```python
from build123d import *

# Parameters (mm, degrees)
SKETCH1_R           = 76.2
BOSS_EXTRUDE1_DEPTH = 40
BOSS_EXTRUDE2_DEPTH = 30
CIRPATTERN1_COUNT   = 10
BOSS_EXTRUDE3_DEPTH = 30
CIRPATTERN2_COUNT   = 10
SKETCH4_R           = 7.9375
CUT_EXTRUDE1_DEPTH  = 41
CUT_EXTRUDE2_DEPTH  = 41
CIRPATTERN3_COUNT   = 8
FILLET4_R           = 5
FILLET5_R           = 5


with BuildPart() as part:
    # Sketch1 → Boss-Extrude1 (new body)
    with BuildSketch(Plane(origin=(0, 0, 0), x_dir=(1, 0, 0), z_dir=(0, 1, 0))):
        Circle(SKETCH1_R)
    extrude(amount=BOSS_EXTRUDE1_DEPTH)

    # Sketch2 → Boss-Extrude2 (add)
    with BuildSketch(Plane(origin=(0, 40, 0), x_dir=(1, 0, 0), z_dir=(0, 1, 0))):
        with BuildLine():
            Line((0, 86.2), (0, 76.2))
            ThreePointArc((0, 76.2), (2.860964701, 76.146272929), (5.717894985, 75.98516748))
            Line((5.717894985, 75.98516748), (2, 86.2))
            Line((2, 86.2), (0, 86.2))
        make_face()
        with BuildLine():
            ThreePointArc((-5.717894985, 75.98516748), (-2.860964701, 76.146272929), (0, 76.2))
            Line((0, 76.2), (0, 86.2))
            Line((0, 86.2), (-2, 86.2))
            Line((-2, 86.2), (-5.717894985, 75.98516748))
        make_face()
    boss_extrude2 = extrude(amount=-BOSS_EXTRUDE2_DEPTH)

    # CirPattern1: Boss-Extrude2 ×10 about axis
    cirpattern1_axis = Axis((0, 0, -0.338660651), (0, 1, 0))
    for i in range(1, CIRPATTERN1_COUNT):
        add(boss_extrude2.rotate(cirpattern1_axis, i * 360 / CIRPATTERN1_COUNT))

    # Sketch3 → Boss-Extrude3 (add)
    with BuildSketch(Plane.XZ):
        with BuildLine():
            Line((24.811616962, 82.515457643), (17.980532935, 74.048230468))
            ThreePointArc((17.980532935, 74.048230468), (20.820375524, 73.300422666), (23.629294983, 72.44374658))
            Line((23.629294983, 72.44374658), (26.73025233, 81.950799937))
            Line((26.73025233, 81.950799937), (24.811616962, 82.515457643))
        make_face()
        with BuildLine():
            Line((26.73025233, 81.950799937), (23.629294983, 72.44374658))
            ThreePointArc((23.629294983, 72.44374658), (26.423605423, 71.471904105), (29.178084826, 70.392324624))
            Line((29.178084826, 70.392324624), (28.648887698, 81.386142232))
            Line((28.648887698, 81.386142232), (26.73025233, 81.950799937))
        make_face()
    boss_extrude3 = extrude(amount=-BOSS_EXTRUDE3_DEPTH)

    # CirPattern2: Boss-Extrude3 ×10 about axis
    cirpattern2_axis = Axis((0.107387074, 0, 0.328898849), (0, 1, 0))
    for i in range(1, CIRPATTERN2_COUNT):
        add(boss_extrude3.rotate(cirpattern2_axis, i * 360 / CIRPATTERN2_COUNT))

    # Sketch4 → Cut-Extrude1 (cut, through all)
    with BuildSketch(Plane(origin=(0, 40, 0), x_dir=(1, 0, 0), z_dir=(0, 1, 0))):
        Circle(SKETCH4_R)
    extrude(amount=-CUT_EXTRUDE1_DEPTH, mode=Mode.SUBTRACT)

    # Sketch5 → Cut-Extrude2 (cut, through all)
    with BuildSketch(Plane(origin=(0, 40, 0), x_dir=(1, 0, 0), z_dir=(0, 1, 0))):
        with BuildLine():
            ThreePointArc((15, 62.217360921), (0, 64), (-15, 62.217360921))
            Line((-15, 62.217360921), (-5, 19.364916731))
            ThreePointArc((-5, 19.364916731), (0, 20), (5, 19.364916731))
            Line((5, 19.364916731), (15, 62.217360921))
        make_face()
    cut_extrude2 = extrude(amount=-CUT_EXTRUDE2_DEPTH, mode=Mode.SUBTRACT)

    # CirPattern3: Cut-Extrude2 ×8 about axis
    cirpattern3_axis = Axis((0, 0, 0), (0, 1, 0))
    for i in range(1, CIRPATTERN3_COUNT):
        add(cut_extrude2.rotate(cirpattern3_axis, i * 360 / CIRPATTERN3_COUNT), mode=Mode.SUBTRACT)

    # Fillet4
    fillet4_edges = [part.edges().sort_by_distance(p)[0] for p in [
        (5, 20, -19.364916731),
        (-5, 20, -19.364916731),
        (15, 20, -62.217360921),
        (-5, 20, 19.364916731),
        (5, 20, 19.364916731),
        (-15, 20, 62.217360921),
        (10.157530032, 20, 17.228597844),
        (17.228597844, 20, 10.157530032),
        (33.387716097, 20, 54.600919533),
        (-19.364916731, 20, -5),
        (-19.364916731, 20, 5),
        (-62.217360921, 20, -15),
        (-17.228597844, 20, 10.157530032),
        (-10.157530032, 20, 17.228597844),
        (-54.600919533, 20, 33.387716097),
        (17.228597844, 20, -10.157530032),
        (10.157530032, 20, -17.228597844),
        (54.600919533, 20, -33.387716097),
        (19.364916731, 20, 5),
        (19.364916731, 20, -5),
        (62.217360921, 20, 15),
        (-10.157530032, 20, -17.228597844),
        (-17.228597844, 20, -10.157530032),
        (-33.387716097, 20, -54.600919533),
    ]]
    fillet(fillet4_edges, radius=FILLET4_R)

    # Fillet5
    fillet5_edges = [part.edges().sort_by_distance(p)[0] for p in [
        (-15, 20, -62.217360921),
        (15, 20, 62.217360921),
        (54.600919533, 20, 33.387716097),
        (-62.217360921, 20, 15),
        (-33.387716097, 20, 54.600919533),
        (33.387716097, 20, -54.600919533),
        (62.217360921, 20, -15),
        (-54.600919533, 20, -33.387716097),
    ]]
    fillet(fillet5_edges, radius=FILLET5_R)


solid = part.part
```
For this review, take the finished solid that the model builds, in its own axes (mm). A direction names the side the tool comes from. Give positions to 0.01 mm unless a question says otherwise; leave off trailing zeros. Write each loop counter-clockwise with the first axis right and the second up, starting at its lowest first coordinate (ties: lowest second). Pieces come first, ordered by that corner, then holes. Notation, with made-up numbers: M -1,38.5 L 15,38.5 A20 ccw 15,48.5 Z; hole C -9.75,-16 d4. An arc over 180 degrees is marked long. Answer as CSV lines item,"result".
1. For faces 1 (the cylindrical face through (-11.882, 19.72, 17.752)), 2 (the flat face through (21.444, 14.79, 78.341)), 3 (the flat face through (80.94, 14.79, -3.69)), list the 3-axis set-ups (+Z, -Z, +X, -X, +Y, -Y) from which the entire face can be reached by the end or side of a thin tool; tool diameter is ignored.
Findings:
face 1,"+Y, -Y"
face 2,"+Z, +Y, -Y"
face 3,"+X, +Y, -Y"
2. For pin 1 (3 mm diameter, centred on x = -17, y = 23, fed in from -Z); pin 2 (5.5 mm diameter, centred on x = 74.5, z = -26.5, fed in from -Y); pin 3 (3 mm diameter, centred on x = 21, y = 27.5, fed in from +Z), all flat-tipped, find the tip position at first contact; note any pin that passes through.
Findings:
pin 1,"stops at z = -74.61"
pin 2,"stops at y = 10"
pin 3,"stops at z = 79.65"
3. Consider section B-B, the plane x = 46. Write out the cut boundary in (y, z).
Findings:
outline,"M 0,-60.75 L 10,-60.75 L 10,-69.06 L 40,-69.06 L 40,-44.5 L 0,-44.5 Z; M 0,-28.04 L 40,-28.04 L 40,-11.22 L 0,-11.22 Z; M 0,11.22 L 40,11.22 L 40,28.04 L 0,28.04 Z; M 0,44.5 L 40,44.5 L 40,68.38 L 10,68.38 L 10,60.75 L 0,60.75 Z"
4. Consider section C-C, the plane y = 6. Count the separate pieces of the cut face and the enclosed holes in it, then the cut area to 3 significant figures.
Findings:
separate pieces,"1"
enclosed holes,"9"
area,"11,800 mm2"
5. Consider section A-A, the plane z = 44. Write out the cut boundary in (x, y).
Findings:
outline,"M -67.02,0 L -46.48,0 L -46.48,40 L -62.21,40 L -62.21,30 L -67.02,30 Z; M -26.8,0 L -10.75,0 L -10.75,40 L -26.8,40 Z; M 10.75,0 L 26.8,0 L 26.8,40 L 10.75,40 Z; M 46.48,0 L 67.48,0 L 67.48,30 L 62.21,30 L 62.21,40 L 46.48,40 Z"
6. Wall thickness on line 1 (X direction, y = 23.5, z = 0); line 2 (Z direction, x = 0, y = 24); line 3 (Z direction, x = -41.5, y = 32): over which ranges is each line inside the solid? List them lowest first.
Findings:
line 1,"x = -85.73 to -64, -20 to -7.94, 7.94 to 20, 64 to 85.97"
line 2,"z = -86.2 to -64, -20 to -7.94, 7.94 to 20, 64 to 85.52"
line 3,"z = -66.02 to -48.72, -25.24 to -10.17, 10.17 to 25.24, 48.72 to 65.34"
